Can you work these out from the model? Positions are in its coordinate system, mm. A direction names the side the tool comes from. Give positions to 0.01 mm unless a question says otherwise; leave off trailing zeros. Loops run counter-clockwise (first coordinate to the right, second up) from the corner with the lowest first, then second, coordinate; pieces in that order, holes last. Notation, with made-up numbers: M -8,56.5 L 20,56.5 A12 cw 20,73.5 Z; hole C 53.5,23 d3. An arc over 180 degrees is marked long. One line per item, written item: value. Start each with the question number.
from build123d import *

# Parameters (mm, degrees)
CROQUIS1_W              = 10
CROQUIS1_H              = 10
CROQUIS1_H_2            = 20.4
CROQUIS1_R              = 2.1
SALIENTE_EXTRUIR1_DEPTH = 3
CROQUIS2_W              = 5
CROQUIS2_H              = 20
SALIENTE_EXTRUIR2_DEPTH = 8
CORTAR_EXTRUIR1_DEPTH   = 4
CROQUIS4_R              = 2.1
CORTAR_EXTRUIR2_DEPTH   = 185.05302625


with BuildPart() as part:
    # Croquis1 → Saliente-Extruir1 (new body)
    # profile 1 of 6: a face of its own
    with BuildSketch(Plane(origin=(0, 0, -124.398862982), x_dir=(-1, 0, 0), z_dir=(0, 0, -1))):
        with Locations((-5, 178.647805519)):
            Rectangle(CROQUIS1_W, CROQUIS1_H)
        with BuildLine():
            ThreePointArc((-7.522554348, 176.84593994), (-7.904499228, 177.217722585), (-8.39233871, 177.432470964))
            ThreePointArc((-8.39233871, 177.432470964), (-9.35, 178.647805519), (-8.39233871, 179.863140073))
            ThreePointArc((-8.39233871, 179.863140073), (-7.904499228, 180.077888452), (-7.522554348, 180.449671097))
            ThreePointArc((-7.522554348, 180.449671097), (-1.9, 178.647805519), (-7.522554348, 176.84593994))
        make_face(mode=Mode.SUBTRACT)
    # profile 2 of 6: a face of its own
    with BuildSketch(Plane(origin=(0, 0, -124.398862982), x_dir=(-1, 0, 0), z_dir=(0, 0, -1))):
        with Locations((-5, 163.447805519)):
            Rectangle(CROQUIS1_W, CROQUIS1_H_2)
    # profile 3 of 6: a face of its own
    with BuildSketch(Plane(origin=(0, 0, -124.398862982), x_dir=(-1, 0, 0), z_dir=(0, 0, -1))):
        with Locations((-5, 148.247805519)):
            Rectangle(CROQUIS1_W, CROQUIS1_H)
        with BuildLine():
            ThreePointArc((-1.9, 148.247805519), (-4.053934061, 145.295694538), (-7.522554348, 146.44593994))
            ThreePointArc((-7.522554348, 146.44593994), (-8.1, 148.247805519), (-7.522554348, 150.049671097))
            ThreePointArc((-7.522554348, 150.049671097), (-4.053934061, 151.199916499), (-1.9, 148.247805519))
        make_face(mode=Mode.SUBTRACT)
    # profile 4 of 6: a face of its own
    with BuildSketch(Plane(origin=(0, 0, -124.398862982), x_dir=(-1, 0, 0), z_dir=(0, 0, -1))):
        with BuildLine():
            ThreePointArc((-7.522554348, 150.049671097), (-8.1, 148.247805519), (-7.522554348, 146.44593994))
            ThreePointArc((-7.522554348, 146.44593994), (-4.053934061, 145.295694538), (-1.9, 148.247805519))
            ThreePointArc((-1.9, 148.247805519), (-4.053934061, 151.199916499), (-7.522554348, 150.049671097))
        make_face()
        with Locations((-5, 148.247805519)):
            Circle(CROQUIS1_R, mode=Mode.SUBTRACT)
    # profile 5 of 6: a face of its own
    with BuildSketch(Plane(origin=(0, 0, -124.398862982), x_dir=(-1, 0, 0), z_dir=(0, 0, -1))):
        with BuildLine():
            ThreePointArc((-7.522554348, 180.449671097), (-8.1, 178.647805519), (-7.522554348, 176.84593994))
            ThreePointArc((-7.522554348, 176.84593994), (-4.053934061, 175.695694538), (-1.9, 178.647805519))
            ThreePointArc((-1.9, 178.647805519), (-4.053934061, 181.599916499), (-7.522554348, 180.449671097))
        make_face()
        with Locations((-5, 178.647805519)):
            Circle(CROQUIS1_R, mode=Mode.SUBTRACT)
    # profile 6 of 6: a face of its own
    with BuildSketch(Plane(origin=(0, 0, -124.398862982), x_dir=(-1, 0, 0), z_dir=(0, 0, -1))):
        with BuildLine():
            ThreePointArc((-8.39233871, 177.432470964), (-7.904499228, 177.217722585), (-7.522554348, 176.84593994))
            ThreePointArc((-7.522554348, 176.84593994), (-8.1, 178.647805519), (-7.522554348, 180.449671097))
            ThreePointArc((-7.522554348, 180.449671097), (-7.904499228, 180.077888452), (-8.39233871, 179.863140073))
            ThreePointArc((-8.39233871, 179.863140073), (-9.35, 178.647805519), (-8.39233871, 177.432470964))
        make_face()
    extrude(amount=SALIENTE_EXTRUIR1_DEPTH)

    # Croquis2 → Saliente-Extruir2 (add)
    with BuildSketch(Plane(origin=(0, 0, -127.398862982), x_dir=(-1, 0, 0), z_dir=(0, 0, -1))):
        with Locations((-2.5, 163.447805519)):
            Rectangle(CROQUIS2_W, CROQUIS2_H)
        with Locations((-7.5, 163.447805519)):
            Rectangle(CROQUIS2_W, CROQUIS2_H)
    extrude(amount=SALIENTE_EXTRUIR2_DEPTH)

    # Croquis3 → Cortar-Extruir1 (cut)
    with BuildSketch(Plane(origin=(0, 0, -135.398862982), x_dir=(-1, 0, 0), z_dir=(0, 0, -1))):
        with BuildLine():
            ThreePointArc((-1.9, 163.447805519), (-2.807968978, 165.63983654), (-5, 166.547805519))
            Line((-5, 166.547805519), (-5, 160.347805519))
            ThreePointArc((-5, 160.347805519), (-2.807968978, 161.255774497), (-1.9, 163.447805519))
        make_face()
        with BuildLine():
            Line((-5, 160.347805519), (-5, 166.547805519))
            ThreePointArc((-5, 166.547805519), (-8.1, 163.447805519), (-5, 160.347805519))
        make_face()
    extrude(amount=-CORTAR_EXTRUIR1_DEPTH, mode=Mode.SUBTRACT)

    # Croquis4 → Cortar-Extruir2 (cut, through all)
    with BuildSketch(Plane(origin=(0, 0, -131.398862982), x_dir=(-1, 0, 0), z_dir=(0, 0, -1))):
        with Locations((-5, 163.447805519)):
            Circle(CROQUIS4_R)
    extrude(amount=-CORTAR_EXTRUIR2_DEPTH, mode=Mode.SUBTRACT)


solid = part.part
Q1. Which directions (+Z, -Z, +X, -X, +Y, -Y) give clear straight access to the entire face, cutting with the end or side of a thin tool? Please do faces 4 (the face through (5, 173.448, -131)), 5 (the face through (7.3, 165.8, -135.399)), 6 (the face through (5, 153.448, -131)).
Q2. If we section it at A-A, the plane y = 163: Write out the boundary of the cut face in (x, z).
Q3. If we mould it in two halves opening along Y, with no side actions, what happens to faces 1 (the face through (7.3, 178.6, -127.399)), 2 (the face through (5, 183.648, -126)), 3 (the face through (4, 161, -131.399))? For each: released by +Y, released by -Y, zero draft, split by the parting line, or undercut.
Q4. If we section it at D-D, the plane z = -126: Write out the boundary of the cut face in (x, y).
Q5. If we section it at B-B, the plane z = -134: Write out the boundary of the cut face in (x, y), plus the area to 3 significant figures.
Q6. If we section it at C-C, the plane x = 9.5: Write out the boundary of the cut face in (y, z), plus the area to 3 significant figures.
Q7. I need wall thicknesses on line 1 along Y through (x, z) = (5, -126.65); line 2 along Y through (x, z) = (5, -128); line 3 along Y through (x, z) = (5, -134.25). Which ranges of each line are inside material? Lowest first, please.
Q8. For P1, Ø4, axis at x = 4.5, z = -132, coming from the +Y side, with a flat end and sliding along its axis, tell me the tip position at first contact or that it passes through.
Response:
1. face 4: -Z, +X, -X, +Y
1. face 5: -Z, +X, -X, +Y, -Y
1. face 6: -Z, +X, -X, -Y
2. outline: M 0,-135.4 L 1.93,-135.4 L 1.93,-131.4 L 2.95,-131.4 L 2.95,-124.4 L 0,-124.4 Z; M 7.05,-131.4 L 8.07,-131.4 L 8.07,-135.4 L 10,-135.4 L 10,-124.4 L 7.05,-124.4 Z
3. face 1: zero draft
3. face 2: released by +Y
3. face 3: undercut
4. outline: M 0,143.25 L 10,143.25 L 10,183.65 L 0,183.65 Z; hole C 5,148.25 d4.2; hole C 5,163.45 d4.2; hole C 5,178.65 d4.2
5. outline: M 0,153.45 L 10,153.45 L 10,173.45 L 0,173.45 Z; hole C 5,163.45 d6.2
5. area: 170 mm^2
6. outline: M 143.25,-127.4 L 153.45,-127.4 L 153.45,-135.4 L 173.45,-135.4 L 173.45,-127.4 L 183.65,-127.4 L 183.65,-124.4 L 143.25,-124.4 Z
6. area: 281 mm^2
7. line 1: 143.25 to 146.15, 150.35 to 161.35, 165.55 to 176.55, 180.75 to 183.65
7. line 2: 153.45 to 161.35, 165.55 to 173.45
7. line 3: 153.45 to 160.35, 166.55 to 173.45
8. P1: y = 173.45
